Autodesk Inventor part; units mm, degrees
ref_plane "YZ Plane" through (0, 0, 0) normal (1, 0, 0) x (0, 1, 0)
ref_plane "XZ Plane" through (0, 0, 0) normal (0, 1, 0) x (-1, 0, 0)
ref_plane "XY Plane" through (0, 0, 0) normal (0, 0, 1) x (1, 0, 0)
sketch "Sketch1" plane through (0, 0, 0) normal (0, 1, 0) x (-1, 0, 0)
  line L0 (-28, -36.5) -> (28, -36.5)
  line L1 (28, -36.5) -> (28, 36.5)
  line L2 (28, 36.5) -> (-28, 36.5)
  line L3 (-28, 36.5) -> (-28, -36.5)
  line L4 (-28, -36.5) -> (28, 36.5) construction
  line L5 (28, -36.5) -> (-28, 36.5) construction
  point P0 (0, 0)
  dimension "d0" = 73
  dimension "d1" = 56
extrude "Extrusion1" add sketch "Sketch1" along normal blind 3
sketch "Sketch3" plane through (0, 0, 0) normal (0, -1, 0) x (1, 0, 0)
  line L0 (-7.3, 4.62) -> (-7.3, 15.74)
  line L1 (-17.51, 4.16) -> (-7.86, 4.16)
  line L2 (-17.51, 15.74) -> (-17.51, 4.62)
  line L3 (-7.86, 16.2) -> (-17.51, 16.2)
  line L4 (-18.35, -24.665) -> (-7.85, -24.665)
  line L5 (-7.35, -24.165) -> (-7.35, -16.165)
  arc A0 (-7.85, -24.665) -> (-7.35, -24.165) centre (-7.85, -24.165) ccw
  arc A1 (-7.35, -16.165) -> (-7.85, -15.665) centre (-7.85, -16.165) ccw
  line L6 (-7.85, -15.665) -> (-18.35, -15.665)
  line L7 (-18.35, -15.665) -> (-18.35, -24.665)
  line L8 (-7.3, 4.62) -> (-7.3, 4.16)
  line L9 (-7.3, 4.16) -> (-7.86, 4.16)
  line L10 (-7.86, 16.2) -> (-7.3, 16.2)
  line L11 (-7.3, 16.2) -> (-7.3, 15.74)
  line L12 (-17.51, 16.2) -> (-17.51, 15.74)
  line L13 (-17.51, 4.16) -> (-17.51, 4.62)
  line L14 (-6.8, 15.74) -> (-6.8, 4.62)
  line L15 (-6.8, 4.62) -> (-6.8, 3.66)
  line L16 (-6.8, 3.66) -> (-7.86, 3.66)
  line L17 (-7.86, 3.66) -> (-18.01, 3.66)
  line L18 (-18.01, 3.66) -> (-18.01, 4.62)
  line L19 (-18.01, 4.62) -> (-18.01, 15.74)
  line L20 (-18.01, 15.74) -> (-18.01, 16.7)
  line L21 (-18.01, 16.7) -> (-7.86, 16.7)
  line L22 (-7.86, 16.7) -> (-6.8, 16.7)
  line L23 (-6.8, 16.7) -> (-6.8, 15.74)
  line L24 (-18.85, -15.165) -> (-7.85, -15.165)
  arc A2 (-6.85, -16.165) -> (-7.85, -15.165) centre (-7.85, -16.165) ccw
  line L25 (-6.85, -16.165) -> (-6.85, -24.165)
  arc A3 (-7.85, -25.165) -> (-6.85, -24.165) centre (-7.85, -24.165) ccw
  line L26 (-7.85, -25.165) -> (-18.85, -25.165)
  line L27 (-18.85, -25.165) -> (-18.85, -15.165)
  dimension "d38" = 0.5
  dimension "d39" = 0.5
extrude "Extrusion3" cut sketch "Sketch3" against normal through all contours L8 L9 L1 L13 L2 L12 L3 L10 L11 L0 | L7 L6 A1 L5 A0 L4 | L14 L15 L16 L17 L18 L19 L20 L21 L22 L23 | L24 A2 L25 A3 L26 L27
sketch "Sketch4" plane through (0, 0, 0) normal (0, -1, 0) x (1, 0, 0)
  circle A0 centre (12, 0) radius 3.5
  line L0 (28, 36.5) -> (28, -36.5)
  point P0 (0, 0)
  dimension "d12" = 7
  dimension "d13" = 16
extrude "Extrusion4" cut sketch "Sketch4" against normal through all
sketch "Sketch7" plane through (0, 0, 0) normal (0, -1, 0) x (1, 0, 0)
  line L0 (-5, 36.5) -> (5, 36.5)
  line L1 (5, 36.5) -> (5, 33.5)
  line L2 (5, 33.5) -> (-5, 33.5)
  line L3 (-5, 33.5) -> (-5, 36.5)
  line L4 (-5, 36.5) -> (5, 33.5) construction
  line L5 (5, 36.5) -> (-5, 33.5) construction
  line L6 (-28, 36.5) -> (28, 36.5)
  line L7 (-5, -36.5) -> (5, -36.5)
  line L8 (5, -36.5) -> (5, -33.5)
  line L9 (5, -33.5) -> (-5, -33.5)
  line L10 (-5, -33.5) -> (-5, -36.5)
  line L11 (-5, -36.5) -> (5, -33.5) construction
  line L12 (5, -36.5) -> (-5, -33.5) construction
  line L13 (28, -36.5) -> (-28, -36.5)
  line L14 (-28, -5) -> (-25, -5)
  line L15 (-25, -5) -> (-25, 5)
  line L16 (-25, 5) -> (-28, 5)
  line L17 (-28, 5) -> (-28, -5)
  line L18 (-28, -5) -> (-25, 5) construction
  line L19 (-25, -5) -> (-28, 5) construction
  line L20 (-28, -36.5) -> (-28, 36.5)
  line L21 (25, -5) -> (28, -5)
  line L22 (28, -5) -> (28, 5)
  line L23 (28, 5) -> (25, 5)
  line L24 (25, 5) -> (25, -5)
  line L25 (25, -5) -> (28, 5) construction
  line L26 (28, -5) -> (25, 5) construction
  line L27 (28, 36.5) -> (28, -36.5)
  point P0 (0, 0)
  point P1 (0, 35)
  point P2 (0, 36.5)
  point P3 (0, -35)
  point P4 (0, -36.5)
  point P5 (-26.5, 0)
  point P6 (26.5, 0)
  dimension "d26" = 10
  dimension "d27" = 3
  dimension "d28" = 10
  dimension "d29" = 3
  dimension "d30" = 3
  dimension "d31" = 10
  dimension "d32" = 3
  dimension "d33" = 10
  dimension "d36" = 36.5
extrude "Extrusion7" cut sketch "Sketch7" against normal through all contours L0 L1 L2 L3 | L16 L15 L14 L17 | L22 L21 L24 L23 | L10 L9 L8 L7
sketch "Sketch9" plane through (0, 0, 0) normal (0, -1, 0) x (1, 0, 0)
  line L0 (25, 5) -> (28, 5)
  line L1 (25, 5) -> (25, 36.5)
  line L2 (5, 36.5) -> (28, 36.5)
  line L3 (25, -5) -> (25, 5)
  line L4 (25, -5) -> (25, -36.5)
  line L5 (28, -36.5) -> (5, -36.5)
  line L6 (28, 36.5) -> (28, 5)
  line L7 (28, -5) -> (25, -5)
  line L8 (28, 5) -> (28, -5)
  line L9 (28, -5) -> (28, -36.5)
  point P0 (0, 0)
extrude "Extrusion8" add sketch "Sketch9" against normal blind 3 contours L0 L8 L7 L3
extrude "Extrusion9" cut sketch "Sketch9" against normal through all contours L1 L2 L6 L0 | L7 L9 L5 L4
sketch "Sketch10" plane through (0, 3, 0) normal (0, 1, 0) x (1, 0, 0)
  line L0 (-5, 36.5) -> (-5, 33.5)
  line L1 (-5, 33.5) -> (5, 33.5)
  line L2 (5, 33.5) -> (5, 36.5)
  line L3 (5, 36.5) -> (25, 36.5)
  line L4 (25, 36.5) -> (25, 5)
  line L5 (25, 5) -> (28, 5)
  line L6 (28, 5) -> (28, -5)
  line L7 (28, -5) -> (25, -5)
  line L8 (25, -5) -> (25, -36.5)
  line L9 (25, -36.5) -> (5, -36.5)
  line L10 (5, -36.5) -> (5, -33.5)
  line L11 (5, -33.5) -> (-5, -33.5)
  line L12 (-5, -33.5) -> (-5, -36.5)
  line L13 (-5, -36.5) -> (-28, -36.5)
  line L14 (-28, -36.5) -> (-28, -5)
  line L15 (-28, -5) -> (-25, -5)
  line L16 (-25, -5) -> (-25, 5)
  line L17 (-25, 5) -> (-28, 5)
  line L18 (-28, 5) -> (-28, 36.5)
  line L19 (-28, 36.5) -> (-5, 36.5)
  circle A0 centre (12, 0) radius 3.5
  line L20 (-7.85, 25.165) -> (-18.85, 25.165)
  line L21 (-18.85, 25.165) -> (-18.85, 15.165)
  line L22 (-18.85, 15.165) -> (-7.85, 15.165)
  arc A1 (-7.85, 15.165) -> (-6.85, 16.165) centre (-7.85, 16.165) ccw
  line L23 (-6.85, 16.165) -> (-6.85, 24.165)
  arc A2 (-6.85, 24.165) -> (-7.85, 25.165) centre (-7.85, 24.165) ccw
  line L24 (-6.8, -16.7) -> (-6.8, -3.66)
  line L25 (-6.8, -3.66) -> (-18.01, -3.66)
  line L26 (-18.01, -3.66) -> (-18.01, -16.7)
  line L27 (-18.01, -16.7) -> (-6.8, -16.7)
  point P0 (0, 0)
properties part number "left"
Geometry: final body of the model. Coordinates: model frame, mm. A direction names the side the tool comes from. Round coordinates to 2 decimals unless told otherwise and drop trailing zeros. Loops run counter-clockwise (first coordinate to the right, second up) from the corner with the lowest first, then second, coordinate; pieces in that order, holes last. Notation, with made-up numbers: (-0.75, 48) - (50.25, 48) arc R23 ccw to (50.25, 67) - close; hole circle Ø8 at (19, -38.75). An arc over 180 degrees is marked (long way). Write each question's results on one line, items separated by ' | '. Start each with the question number.
1) Mould query, pull axis X, two halves, no side actions, for faces 5 (the face through (25, 1, 21)), 6 (the face through (15, 1, 36.5)), 7 (the face through (0, 1, 33.5)). Classes: released by +X, released by -X, zero draft, split by the parting line, or undercut.
2) Line query: probe 1 along Z at (x, y) = (-17, 0.75) (3 decimals); probe 2 along X at (y, z) = (1.3, 9); probe 3 along Z at (x, y) = (12, 0.9). Output: solid intervals per line, ascending. Write a range as [from, to].
3) Cut plane C-C on x = 10. Return loops of the section in (y, z), then the cut area to 3 significant figures.
4) First-contact query: P1, Ø0.9, axis at x = 26.5, y = 2, coming from the +Z side; P2, Ø1.5, axis at y = 1, z = -34.5, coming from the +X side. Flat tips, straight axial feed; report the tip coordinate or a pass-through.
5) Cut plane D-D on z = 24.5. Return loops of the section in (x, y), then the cut area to 3 significant figures.
6) Cut plane A-A on z = 0. Return loops of the section in (x, y).
7) Cut plane B-B on y = 2.4. Count the separate pieces of the cut face and the enclosed holes in it, then the cut area to 3 significant figures.
8) Access query for faces 1 (the face through (26, 1, 5)), 2 (the face through (5, 1, 35)), 3 (the face through (-25, 1, 0)), 4 (the face through (-12, 1, 3.66)). Directions: +Z, -Z, +X, -X, +Y, -Y. A direction counts if a zero-diameter tool reaches every point of the face in a straight line with its end or side. Return the directions, or none.
Verdict:
1) face 5: released by +X | face 6: zero draft | face 7: undercut
2) probe 1: z = [-36.5, -25.165], [-15.165, 3.66], [16.7, 36.5] | probe 2: x = [-28, -18.01], [-6.8, 25] | probe 3: z = [-36.5, -3.5], [3.5, 36.5]
3) outline: (0, -36.5) - (3, -36.5) - (3, -2.87) - (0, -2.87) - close; (0, 2.87) - (3, 2.87) - (3, 36.5) - (0, 36.5) - close | area: 202 mm2
4) P1: stops at z = 5 | P2: stops at x = 25
5) outline: (-28, 0) - (25, 0) - (25, 3) - (-28, 3) - close | area: 159 mm2
6) outline: (-25, 0) - (8.5, 0) - (8.5, 3) - (-25, 3) - close; (15.5, 0) - (28, 0) - (28, 3) - (15.5, 3) - close
7) separate pieces: 1 | enclosed holes: 3 | area: 3,500 mm2
8) face 1: +Z, +X, +Y, -Y | face 2: +Z, +Y, -Y | face 3: -X, +Y, -Y | face 4: +Y, -Y
